Here's how the part is built. I have some questions about the finished solid (model axes, mm). A direction names the side the tool comes from. Round coordinates to 2 decimals unless told otherwise and drop trailing zeros. Order: outer loops, then holes, each group sorted by start corner. A loop starts at its lowest first (then second) coordinate and runs counter-clockwise, first axis right, second up. Notation, with made-up numbers: M -4.75,-9.5 L 13.25,-9.5 A21 ccw 13.25,5.5 Z; hole C 80,-22 d5. An arc over 180 degrees is marked long. Write item = value, one per line. Start each with the question number.
Item 1: I want a section at A-A, the plane x = -4.5. List the corners of the cut face in (y, z) for me.
Item 2: We'd pull the mould along Z, two halves only. Please class faces 4 (the face through (-41, 4.415, 174)), 5 (the face through (-5, -5, 0)), 6 (the face through (25.052, -8, 66)): pulls with the +Z half, pulls with the -Z half, needs draft (parallel to the pull), parting line crosses it, or undercut.
Item 3: I want a section at B-B, the plane z = 280. List the corners of the cut face in (x, y) for me.
Item 4: Please list where these lines run through material, in increasing order: L1, parallel to Z at x = 23, y = -12.5; L2, parallel to Z at x = 12.5, y = 2.5; L3, parallel to X at y = -6.5, z = 100.5.
Item 5: For faces 1 (the face through (-4, 1, 4)), 2 (the face through (-45.832, -6, 173)), 3 (the face through (-35.25, -8, 100)), which set-ups out of +Z, -Z, +X, -X, +Y, -Y let a thin tool reach every point of the face, with its end or its side?
Item 6: I'm going to push a flat-ended pin straight in: P1, Ø3, axis at x = 11, y = 1, coming from the -Z side. Where does the tip first touch, or does it pass through?
```python
from build123d import *

# Parameters (mm, degrees)
SKETCH_1_W          = 80
SKETCH_1_H          = 20
EXTRUDE_1_DEPTH     = 350
SKETCH_2_W          = 67.355648201
SKETCH_2_H          = 6
CUT_EXTRUDE_1_DEPTH = 351
SKETCH_3_W          = 60.301963697
SKETCH_3_H          = 16
CUT_EXTRUDE_2_DEPTH = 15
SKETCH_4_W          = 67.355648201
SKETCH_4_H          = 6
EXTRUDE_2_DEPTH     = 4
SKETCH_5_W          = 67.355648201
SKETCH_5_H          = 6
EXTRUDE_3_DEPTH     = 4


with BuildPart() as part:
    # 草图1 → 凸台-拉伸1 (new body)
    with BuildSketch(Plane.XY):
        with Locations((-5.831622177, -5.58518109)):
            Rectangle(SKETCH_1_W, SKETCH_1_H)
    extrude(amount=EXTRUDE_1_DEPTH)

    # 草图2 → 切除-拉伸1 (cut, through all)
    with BuildSketch(Plane.XY.offset(350)):
        with Locations((-4.554011248, 1.41481891)):
            Rectangle(SKETCH_2_W, SKETCH_2_H)
    extrude(amount=-CUT_EXTRUDE_1_DEPTH, mode=Mode.SUBTRACT)

    # 草图3 → 切除-拉伸2 (cut, through all)
    with BuildSketch(Plane(origin=(0, -1.58518109, 0), x_dir=(1, 0, 0), z_dir=(0, 1, 0))):
        with Locations((-5.099475916, -65.71132948)):
            Rectangle(SKETCH_3_W, SKETCH_3_H)
        with Locations((-5.099475916, -99.71132948)):
            Rectangle(SKETCH_3_W, SKETCH_3_H)
    extrude(amount=-CUT_EXTRUDE_2_DEPTH, mode=Mode.SUBTRACT)

    # 草图4 → 凸台-拉伸2 (add)
    with BuildSketch(Plane.XY.offset(350)):
        with Locations((-4.554011248, 1.41481891)):
            Rectangle(SKETCH_4_W, SKETCH_4_H)
    extrude(amount=-EXTRUDE_2_DEPTH)

    # 草图5 → 凸台-拉伸3 (add)
    with BuildSketch(Plane(origin=(0, 0, 0), x_dir=(-1, 0, 0), z_dir=(0, 0, -1))):
        with Locations((4.554011248, 1.41481891)):
            Rectangle(SKETCH_5_W, SKETCH_5_H)
    extrude(amount=-EXTRUDE_3_DEPTH)


solid = part.part
```
Filled in:
q1.outline = M -15.59,0 L 4.41,0 L 4.41,4 L -1.59,4 L -1.59,57.71 L -15.59,57.71 Z; M -15.59,73.71 L -1.59,73.71 L -1.59,91.71 L -15.59,91.71 Z; M -15.59,107.71 L -1.59,107.71 L -1.59,346 L 4.41,346 L 4.41,350 L -15.59,350 Z
q2.face_4 = needs draft
q2.face_5 = pulls with the -Z half
q2.face_6 = undercut
q3.outline = M -45.83,-15.59 L 34.17,-15.59 L 34.17,4.41 L 29.12,4.41 L 29.12,-1.59 L -38.23,-1.59 L -38.23,4.41 L -45.83,4.41 Z
q4.L1 = 0 to 57.71, 73.71 to 91.71, 107.71 to 350
q4.L2 = 0 to 4, 346 to 350
q4.L3 = -45.83 to -35.25, 25.05 to 34.17
q5.face_1 = +Y
q5.face_2 = +Z, -Z, -X, +Y, -Y
q5.face_3 = +Y, -Y
q6.P1 = 0
